Autodesk Fusion 360 part; units mm, degrees
sketch "Skizze1" plane through (0, 0, 0) normal (0, 0, 1) x (1, 0, 0)
  circle A0 centre (0, 0) radius 3
  circle A1 centre (0, 0) radius 1.5
  dimension "d1" = 6
  dimension "d2" = 3
extrude "Extrusion1" add sketch "Skizze1" along normal blind 5
extrude "Extrusion2" add sketch "Skizze1" along normal blind 6.2 contours A1
sketch "Skizze2" plane through (0, 0, 0) normal (0, 0, 1) x (1, 0, 0)
  line L0 (-5, 5) -> (5, 5)
  line L1 (5, 5) -> (5, -5)
  line L2 (5, -5) -> (-5, -5)
  line L3 (-5, -5) -> (-5, 5)
  dimension "d9" = 10
extrude "Extrusion3" add sketch "Skizze2" along normal blind 0.5
equation "d5 = 5 mm + ( 0.12 * 10 ) * 1 mm"
For this review, take the finished solid that the model builds, in its own axes (mm). A direction names the side the tool comes from. Round coordinates to 2 decimals unless told otherwise and drop trailing zeros. Order: outer loops, then holes, each group sorted by start corner. A loop starts at its lowest first (then second) coordinate and runs counter-clockwise, first axis right, second up. Notation, with made-up numbers: M 43,33 L 100,33 A16 ccw 100,63 Z; hole C 32.25,27 d9. An arc over 180 degrees is marked long. Use a Markdown table: item, result. Add a question column.
Item 1: Tool access review of faces 4 (the flat face through (2.2, 2.3, 0.5)), 5 (the flat face through (0, 0, 6.2)): name each direction out of +Z, -Z, +X, -X, +Y, -Y from which nothing blocks a thin tool from reaching the whole face with its end or side.
Item 2: To check wall thickness, follow line 1 along Z through (x, y) = (4.5, 3); line 2 along Z through (x, y) = (-2.75, 1); line 3 along Y through (x, z) = (1, 4.25). State the ranges of each line that lie inside material, in increasing order.
Item 3: Insertion check: pin 1 (3 mm diameter, centred on y = 2.5, z = 3, fed in from -X); pin 2 (1 mm diameter, centred on x = 0, z = 3, fed in from -Y); pin 3 (1.5 mm diameter, centred on y = -3, z = 1, fed in from +X); pin 4 (1.5 mm diameter, centred on x = -3.5, z = 4.5, fed in from -Y). Each pin has a flat end and moves straight along its axis. Give the tip position at first contact, or say it passes through.
Item 4: Mouldability with a two-part tool opening along Z and no side actions: class faces 1 (the cylindrical face through (-1.5, -0.07, 5.59)), 2 (the flat face through (0, 0, 0)), 3 (the flat face through (1.3, -1.3, 5)) as released by +Z, released by -Z, zero draft, split by the parting line, or undercut.
Item 5: Add section D-D, the plane y = 2. Give the boundary of the cut face in (x, z), then the cut area to 3 significant figures.
Item 6: Add section A-A, the plane x = 0. Give the boundary of the cut face in (y, z).
Item 7: Add section C-C, the plane z = 2.75. Give the boundary of the cut face in (x, y), then the cut area to 3 significant figures.
Item 8: Add section B-B, the plane y = 0.5. Give the boundary of the cut face in (x, z), then the cut area to 3 significant figures.
Geometry results:
| question | item | result |
|---|---|---|
| 1 | face 4 | +Z |
| 1 | face 5 | +Z, +X, -X, +Y, -Y |
| 2 | line 1 | z = 0 to 0.5 |
| 2 | line 2 | z = 0 to 5 |
| 2 | line 3 | y = -2.83 to 2.83 |
| 3 | pin 1 | stops at x = -2.83 |
| 3 | pin 2 | stops at y = -3 |
| 3 | pin 3 | stops at x = 5 |
| 3 | pin 4 | stops at y = -1.2 |
| 4 | face 1 | zero draft |
| 4 | face 2 | released by -Z |
| 4 | face 3 | released by +Z |
| 5 | outline | M -5,0 L 5,0 L 5,0.5 L 2.24,0.5 L 2.24,5 L -2.24,5 L -2.24,0.5 L -5,0.5 Z |
| 5 | area | 25.1 mm² |
| 6 | outline | M -5,0 L 5,0 L 5,0.5 L 3,0.5 L 3,5 L 1.5,5 L 1.5,6.2 L -1.5,6.2 L -1.5,5 L -3,5 L -3,0.5 L -5,0.5 Z |
| 7 | outline | C 0,0 d6 |
| 7 | area | 28.3 mm² |
| 8 | outline | M -5,0 L 5,0 L 5,0.5 L 2.96,0.5 L 2.96,5 L 1.41,5 L 1.41,6.2 L -1.41,6.2 L -1.41,5 L -2.96,5 L -2.96,0.5 L -5,0.5 Z |
| 8 | area | 35.0 mm² |
